from build123d import *

# Parameters (mm, degrees)
BOSS_EXTRUDE1_DEPTH            = 8
SKETCH3_R                      = 12.75
CUT_EXTRUDE1_DEPTH             = 8
SKETCH5_W                      = 139
SKETCH5_H                      = 67
BOSS_EXTRUDE2_DEPTH            = 109
CUT_EXTRUDE2_START             = 10
SKETCH6_R                      = 26.5
CUT_EXTRUDE2_DEPTH             = 16
CUT_EXTRUDE3_REACH             = 169.909
SKETCH7_R                      = 6.5
CUT_EXTRUDE4_REACH             = 169.909
SKETCH10_W                     = 139
SKETCH10_H                     = 0.25
CUT_EXTRUDE8_START             = 36
SKETCH15_R                     = 32.5
CUT_EXTRUDE8_DEPTH             = 20
CUT_EXTRUDE9_DEPTH             = 216.172605134
CUT_EXTRUDE9_DEPTH_BACK        = 216.172605134
SKETCH16_W                     = 20
SKETCH16_H                     = 20
CUT_EXTRUDE10_START            = 56
SKETCH17_R                     = 26.5
CUT_EXTRUDE10_DEPTH            = 26
BOSS_EXTRUDE6_START            = 56
SKETCH20_W                     = 139
SKETCH20_H                     = 66.75
BOSS_EXTRUDE6_DEPTH            = 10
CUT_EXTRUDE12_REACH            = 169.909
SKETCH21_R                     = 13
FILLET1_R                      = 5
FILLET2_R                      = 5
CUT_EXTRUDE13_DEPTH            = 168.909201654
CUT_EXTRUDE13_DEPTH_BACK       = 17
CUT_EXTRUDE13_START            = 109
SKETCH22_R                     = 9
BOSS_EXTRUDE7_DEPTH            = 10
SKETCH24_W                     = 30
SKETCH24_H                     = 30
CUT_EXTRUDE14_DEPTH            = 109
CUT_EXTRUDE15_DEPTH            = 196.139052985
CUT_EXTRUDE15_DEPTH_BACK       = 196.139052985
SKETCH25_W                     = 30
SKETCH25_H                     = 30
SKETCH25_W_2                   = 43
CUT_EXTRUDE16_DEPTH            = 216.172605134
CUT_EXTRUDE16_DEPTH_BACK       = 12
SKETCH29_W                     = 15
SKETCH29_H                     = 7.5
SKETCH30_W                     = 15
SKETCH30_H                     = 7.5
CUT_EXTRUDE17_DEPTH            = 12
SKETCH31_W                     = 7.5
SKETCH31_H                     = 16.75
CUT_EXTRUDE18_DEPTH            = 7
SKETCH32_W                     = 7.5
SKETCH32_H                     = 16.75
CUT_EXTRUDE19_DEPTH            = 7
SKETCH38_W                     = 20
SKETCH38_H                     = 20
CUT_EXTRUDE20_DEPTH            = 168.914598829
FILLET3_R                      = 2
FILLET4_R                      = 2
SKETCH39_W                     = 79
SKETCH39_H                     = 5.5
CUT_EXTRUDE21_DEPTH            = 36
CBORE_FOR_M4_SHCS1_D           = 4.5
CBORE_FOR_M4_SHCS1_CBORE_D     = 8
CBORE_FOR_M4_SHCS1_CBORE_DEPTH = 4
CUT_EXTRUDE22_DEPTH            = 174.20941083
CUT_EXTRUDE22_DEPTH_BACK       = 174.20941083
SKETCH43_W                     = 70
SKETCH43_H                     = 40


with BuildPart() as part:
    # Sketch2 → Boss-Extrude1 (new body)
    with BuildSketch(Plane.XY):
        with BuildLine():
            Line((-57.5, 60), (-57.5, 50))
            ThreePointArc((-57.5, 50), (-59.696699141, 44.696699141), (-65, 42.5))
            Line((-65, 42.5), (-75, 42.5))
            ThreePointArc((-75, 42.5), (-80.303300859, 40.303300859), (-82.5, 35))
            Line((-82.5, 35), (-82.5, -90))
            ThreePointArc((-82.5, -90), (-80.303300859, -95.303300859), (-75, -97.5))
            Line((-75, -97.5), (75, -97.5))
            ThreePointArc((75, -97.5), (80.303300859, -95.303300859), (82.5, -90))
            Line((82.5, -90), (82.5, 35))
            ThreePointArc((82.5, 35), (80.303300859, 40.303300859), (75, 42.5))
            Line((75, 42.5), (65, 42.5))
            ThreePointArc((65, 42.5), (59.696699141, 44.696699141), (57.5, 50))
            Line((57.5, 50), (57.5, 60))
            ThreePointArc((57.5, 60), (55.303300859, 65.303300859), (50, 67.5))
            Line((50, 67.5), (-50, 67.5))
            ThreePointArc((-50, 67.5), (-55.303300859, 65.303300859), (-57.5, 60))
        make_face()
    extrude(amount=-BOSS_EXTRUDE1_DEPTH)

    # Sketch3 → Cut-Extrude1 (cut)
    with BuildSketch(Plane.XY):
        with Locations((0, -20)):
            Circle(SKETCH3_R)
    extrude(amount=-CUT_EXTRUDE1_DEPTH, mode=Mode.SUBTRACT)

    # Sketch5 → Boss-Extrude2 (add)
    with BuildSketch(Plane(origin=(0, 0, -8), x_dir=(-1, 0, 0), z_dir=(0, 0, -1))):
        with Locations((0, -53.5)):
            Rectangle(SKETCH5_W, SKETCH5_H)
    extrude(amount=BOSS_EXTRUDE2_DEPTH)

    # Sketch6 → Cut-Extrude2 (cut)
    with BuildSketch(Plane(origin=(0, 0, -8), x_dir=(-1, 0, 0), z_dir=(0, 0, -1)).offset(CUT_EXTRUDE2_START)):
        with Locations((0, -20)):
            Circle(SKETCH6_R)
    extrude(amount=CUT_EXTRUDE2_DEPTH, mode=Mode.SUBTRACT)

    # Cut-Extrude3: up to this face of the body (flat: up to its plane)
    cut_extrude3_end = Plane(part.part.faces().sort_by_distance((0, -53.5, -117))[0])
    # Sketch7 → Cut-Extrude3 (cut, up to the picked face)
    with BuildSketch(Plane(origin=(0, 0, -8), x_dir=(-1, 0, 0), z_dir=(0, 0, -1)), mode=Mode.PRIVATE) as cut_extrude3_sk1:
        with Locations((0, -20)):
            Circle(SKETCH7_R)
    cut_extrude3_tool1 = split(extrude(cut_extrude3_sk1.sketch, amount=CUT_EXTRUDE3_REACH, mode=Mode.PRIVATE), bisect_by=cut_extrude3_end, keep=Keep.BOTH, mode=Mode.PRIVATE)
    add(cut_extrude3_tool1.solids().sort_by(Axis((0, -20, -8), (0, 0, -1)))[0], mode=Mode.SUBTRACT)

    # Cut-Extrude4: up to this face of the body (flat: up to its plane)
    cut_extrude4_end = Plane(part.part.faces().sort_by_distance((0, -53.720640565, -117))[0])
    # Sketch10 → Cut-Extrude4 (cut, up to the picked face)
    with BuildSketch(Plane(origin=(0, 0, -8), x_dir=(-1, 0, 0), z_dir=(0, 0, -1)), mode=Mode.PRIVATE) as cut_extrude4_sk1:
        with Locations((0, -20.125)):
            Rectangle(SKETCH10_W, SKETCH10_H)
    cut_extrude4_tool1 = split(extrude(cut_extrude4_sk1.sketch, amount=CUT_EXTRUDE4_REACH, mode=Mode.PRIVATE), bisect_by=cut_extrude4_end, keep=Keep.BOTH, mode=Mode.PRIVATE)
    add(cut_extrude4_tool1.solids().sort_by(Axis((0, -20.125, -8), (0, 0, -1)))[0], mode=Mode.SUBTRACT)

    # Sketch15 → Cut-Extrude8 (cut)
    with BuildSketch(Plane(origin=(0, 0, -8), x_dir=(-1, 0, 0), z_dir=(0, 0, -1)).offset(CUT_EXTRUDE8_START)):
        with Locations((0, -20)):
            Circle(SKETCH15_R)
    extrude(amount=CUT_EXTRUDE8_DEPTH, mode=Mode.SUBTRACT)

    # Sketch16 → Cut-Extrude9 (cut, two sides: drawn at the far end of the back side and taken through both)
    with BuildSketch(Plane(origin=(69.5, 0, 0), x_dir=(0, 0, -1), z_dir=(1, 0, 0)).offset(-CUT_EXTRUDE9_DEPTH_BACK)):
        with Locations((54, -30.25)):
            Rectangle(SKETCH16_W, SKETCH16_H)
    extrude(amount=CUT_EXTRUDE9_DEPTH + CUT_EXTRUDE9_DEPTH_BACK, mode=Mode.SUBTRACT)

    # Sketch17 → Cut-Extrude10 (cut)
    with BuildSketch(Plane(origin=(0, 0, -8), x_dir=(-1, 0, 0), z_dir=(0, 0, -1)).offset(CUT_EXTRUDE10_START)):
        with Locations((0, -20)):
            Circle(SKETCH17_R)
    extrude(amount=CUT_EXTRUDE10_DEPTH, mode=Mode.SUBTRACT)

    # Sketch20 → Boss-Extrude6 (add)
    with BuildSketch(Plane(origin=(0, 0, -8), x_dir=(-1, 0, 0), z_dir=(0, 0, -1)).offset(BOSS_EXTRUDE6_START)):
        with Locations((0, -53.625)):
            Rectangle(SKETCH20_W, SKETCH20_H)
    extrude(amount=BOSS_EXTRUDE6_DEPTH)

    # Cut-Extrude12: up to this face of the body (flat: up to its plane)
    cut_extrude12_end = Plane(part.part.faces().sort_by_distance((0, -31.382164936, -74))[0])
    # Sketch21 → Cut-Extrude12 (cut, up to the picked face)
    with BuildSketch(Plane(origin=(0, 0, -8), x_dir=(-1, 0, 0), z_dir=(0, 0, -1)), mode=Mode.PRIVATE) as cut_extrude12_sk1:
        with Locations((0, -20)):
            Circle(SKETCH21_R)
    cut_extrude12_tool1 = split(extrude(cut_extrude12_sk1.sketch, amount=CUT_EXTRUDE12_REACH, mode=Mode.PRIVATE), bisect_by=cut_extrude12_end, keep=Keep.BOTH, mode=Mode.PRIVATE)
    add(cut_extrude12_tool1.solids().sort_by(Axis((0, -20, -8), (0, 0, -1)))[0], mode=Mode.SUBTRACT)

    # Fillet1
    fillet1_edges = [part.edges().sort_by_distance(p)[0] for p in [
        (25.420218331, -40.25, -54),
    ]]
    fillet(fillet1_edges, radius=FILLET1_R)

    # Fillet2
    fillet2_edges = [part.edges().sort_by_distance(p)[0] for p in [
        (-25.420218331, -40.25, -54),
    ]]
    fillet(fillet2_edges, radius=FILLET2_R)

    # Sketch22 → Cut-Extrude13 (cut, two sides: drawn at the far end of the back side and taken through both)
    with BuildSketch(Plane(origin=(0, 0, -8), x_dir=(-1, 0, 0), z_dir=(0, 0, -1)).offset(CUT_EXTRUDE13_START - CUT_EXTRUDE13_DEPTH_BACK)):
        with Locations((0, -20)):
            Circle(SKETCH22_R)
    extrude(amount=CUT_EXTRUDE13_DEPTH + CUT_EXTRUDE13_DEPTH_BACK, mode=Mode.SUBTRACT)

    # Sketch23 → Boss-Extrude7 (add)
    with BuildSketch(Plane(origin=(0, 0, -117), x_dir=(-1, 0, 0), z_dir=(0, 0, -1))):
        with BuildLine():
            Line((-8.996527108, -20.25), (-6.495190528, -20.25))
            ThreePointArc((-6.495190528, -20.25), (0, -26.5), (6.495190528, -20.25))
            Line((6.495190528, -20.25), (8.996527108, -20.25))
            ThreePointArc((8.996527108, -20.25), (0, -29), (-8.996527108, -20.25))
        make_face()
    extrude(amount=-BOSS_EXTRUDE7_DEPTH)

    # Sketch24 → Cut-Extrude14 (cut)
    with BuildSketch(Plane(origin=(0, 0, -117), x_dir=(-1, 0, 0), z_dir=(0, 0, -1))):
        with Locations((-54.5, -72)):
            Rectangle(SKETCH24_W, SKETCH24_H)
        with Locations((54.5, -72)):
            Rectangle(SKETCH24_W, SKETCH24_H)
    extrude(amount=-CUT_EXTRUDE14_DEPTH, mode=Mode.SUBTRACT)

    # Sketch25 → Cut-Extrude15 (cut, two sides: drawn at the far end of the back side and taken through both)
    with BuildSketch(Plane(origin=(39.5, 0, 0), x_dir=(0, 0, -1), z_dir=(1, 0, 0)).offset(-CUT_EXTRUDE15_DEPTH_BACK)):
        with Locations((23, -72)):
            Rectangle(SKETCH25_W, SKETCH25_H)
        with Locations((95.5, -72)):
            Rectangle(SKETCH25_W_2, SKETCH25_H)
    extrude(amount=CUT_EXTRUDE15_DEPTH + CUT_EXTRUDE15_DEPTH_BACK, mode=Mode.SUBTRACT)

    # Sketch29 → Cut-Extrude16 (cut, two sides: drawn at the far end of the back side and taken through both)
    with BuildSketch(Plane(origin=(69.5, 0, 0), x_dir=(0, 0, -1), z_dir=(1, 0, 0)).offset(-CUT_EXTRUDE16_DEPTH_BACK)):
        with Locations((36.5, -24)):
            Rectangle(SKETCH29_W, SKETCH29_H)
        with Locations((71.5, -24)):
            Rectangle(SKETCH29_W, SKETCH29_H)
    extrude(amount=CUT_EXTRUDE16_DEPTH + CUT_EXTRUDE16_DEPTH_BACK, mode=Mode.SUBTRACT)

    # Sketch30 → Cut-Extrude17 (cut)
    with BuildSketch(Plane.ZY.offset(69.5)):
        with Locations((-36.5, -24)):
            Rectangle(SKETCH30_W, SKETCH30_H)
        with Locations((-71.5, -24)):
            Rectangle(SKETCH30_W, SKETCH30_H)
    extrude(amount=-CUT_EXTRUDE17_DEPTH, mode=Mode.SUBTRACT)

    # Sketch31 → Cut-Extrude18 (cut)
    with BuildSketch(Plane.ZY.offset(69.5)):
        with Locations((-54, -48.625)):
            Rectangle(SKETCH31_W, SKETCH31_H)
    extrude(amount=-CUT_EXTRUDE18_DEPTH, mode=Mode.SUBTRACT)

    # Sketch32 → Cut-Extrude19 (cut)
    with BuildSketch(Plane(origin=(69.5, 0, 0), x_dir=(0, 0, -1), z_dir=(1, 0, 0))):
        with Locations((54, -48.625)):
            Rectangle(SKETCH32_W, SKETCH32_H)
    extrude(amount=-CUT_EXTRUDE19_DEPTH, mode=Mode.SUBTRACT)

    # Sketch38 → Cut-Extrude20 (cut, through all)
    with BuildSketch(Plane(origin=(0, -20.25, 0), x_dir=(1, 0, 0), z_dir=(0, 1, 0))):
        with Locations((59.5, 107)):
            Rectangle(SKETCH38_W, SKETCH38_H)
        with Locations((-59.5, 107)):
            Rectangle(SKETCH38_W, SKETCH38_H)
    extrude(amount=-CUT_EXTRUDE20_DEPTH, mode=Mode.SUBTRACT)

    # Fillet3
    fillet3_edges = [part.edges().sort_by_distance(p)[0] for p in [
        (62.5, -57, -54),
    ]]
    fillet(fillet3_edges, radius=FILLET3_R)

    # Fillet4
    fillet4_edges = [part.edges().sort_by_distance(p)[0] for p in [
        (-62.5, -57, -54),
    ]]
    fillet(fillet4_edges, radius=FILLET4_R)

    # Sketch39 → Cut-Extrude21 (cut)
    with BuildSketch(Plane(origin=(0, 0, -74), x_dir=(-1, 0, 0), z_dir=(0, 0, -1))):
        with Locations((0, -84.25)):
            Rectangle(SKETCH39_W, SKETCH39_H)
    extrude(amount=-CUT_EXTRUDE21_DEPTH, mode=Mode.SUBTRACT)

    # CBORE for M4 SHCS1 (through all)
    with Locations(Plane.XY):
        with Locations((-75, 35), (-50, 35), (-50, 60), (-25, 60), (0, 60), (25, 60), (50, 60), (50, 35), (75, 35), (-75, -90), (-50, -90), (-25, -90), (0, -90), (25, -90), (50, -90), (75, -90)):
            CounterBoreHole(CBORE_FOR_M4_SHCS1_D / 2, CBORE_FOR_M4_SHCS1_CBORE_D / 2, CBORE_FOR_M4_SHCS1_CBORE_DEPTH)

    # Sketch43 → Cut-Extrude22 (cut, two sides: drawn at the far end of the back side and taken through both)
    with BuildSketch(Plane.XY.offset(-CUT_EXTRUDE22_DEPTH_BACK)):
        with Locations((0, 32.5)):
            Rectangle(SKETCH43_W, SKETCH43_H)
    extrude(amount=CUT_EXTRUDE22_DEPTH + CUT_EXTRUDE22_DEPTH_BACK, mode=Mode.SUBTRACT)


solid = part.part
Verification items for the finished model (mm, model axes). A direction names the side the tool comes from. Give positions to 0.01 mm unless a question says otherwise; leave off trailing zeros. Loops run counter-clockwise (first coordinate to the right, second up) from the corner with the lowest first, then second, coordinate; pieces in that order, holes last.
1. Cross-section at B-B on x = 0. Count the separate pieces of the cut face and the enclosed holes in it, and give its area (3 significant figures).
Derived:
separate pieces: 5
enclosed holes: 0
area: 3,530 mm2
2. Tool access check on faces 5 (the cylindrical face through (-50.867, 56.095, -1.972)), 6 (the flat face through (-49, -40.25, -54)), 7 (the flat face through (63, -24, -29)), 8 (the flat face through (-60, -38, -97)). Record the directions out of +Z, -Z, +X, -X, +Y, -Y that give a thin tool (end or side, any length) a straight path to the whole face; none if there is none.
Derived:
face 5: +Z
face 6: +X, -X, +Y
face 7: +X, +Y
face 8: -Z, -X, +Y, -Y
3. Release check for a two-part mould opening along X. For faces 1 (the flat face through (-1, -38, -117)), 2 (the flat face through (57.5, -24, -71)), 3 (the flat face through (-39.5, -69, -56)), 4 (the cylindrical face through (51.786, 58.631, -6.028)) record: +X half, -X half, draft (parallel to the pull), parting line (faces both ways), or undercut.
Derived:
face 1: draft
face 2: +X half
face 3: -X half
face 4: undercut
4. Cross-section at A-A on z = -103. Record the cut outline in (x, y).
Derived:
outline: (-49.5, -57) - (49.5, -57) - (49.5, -20.25) - (9, -20.25) arc R9 cw to (-9, -20.25) - (-49.5, -20.25) - close
5. Go/stop test with flat-tipped pins: P1, Ø4, axis at x = -61, y = -23.5, coming from the -Z side; P2, Ø4, axis at x = -1, y = 59, coming from the +Z side; P3, Ø6, axis at y = -47.5, z = -110.5, coming from the +X side. Record where each tip stops, or that it passes through.
Derived:
P1: stops at z = -97
P2: stops at z = -4
P3: stops at x = 49.5
6. Material ranges on probe 1 along Y at (x, z) = (-25, -1.5); probe 2 along Y at (x, z) = (-50, -0.95); probe 3 along Y at (x, z) = (0, -6), recorded low to high.
Derived:
probe 1: y = -97.5 to -94, -86 to 12.5, 52.5 to 56, 64 to 67.5
probe 2: y = -97.5 to -94, -86 to 31, 39 to 56, 64 to 67.5
probe 3: y = -97.5 to -92.25, -87.75 to -32.75, -7.25 to 12.5, 52.5 to 57.75, 62.25 to 67.5
